The model under review builds one solid part; all positions refer to its coordinate system, in mm. Face numbers are marked on the shaded views. A direction names the side the tool comes from. Round coordinates to 2 decimals unless told otherwise and drop trailing zeros. Loops run counter-clockwise (first coordinate to the right, second up) from the corner with the lowest first, then second, coordinate; pieces in that order, holes last. Notation, with made-up numbers: M 42.25,59 L 51.25,59 A21 ccw 51.25,74 Z; hole C -2,-37 d11. An arc over 180 degrees is marked long. Answer as a JSON object with one key per item and string values. Group by question number.
Item 1: To check wall thickness, follow line 1 (X direction, y = -8, z = 8); line 2 (X direction, y = 37.5, z = 4.25); line 3 (Y direction, x = 5, z = 5.5). State the ranges of each line that lie inside material, in increasing order.
Item 2: Consider section B-B (y = -7). Give the boundary of the cut face in (x, z).
Item 3: Consider section C-C (x = -2). Give the boundary of the cut face in (y, z).
Item 4: Consider section A-A (z = 2.5). Give the boundary of the cut face in (x, y) (1 decimal).
Item 5: Insertion check: P1, Ø1.1, axis at y = -24.75, z = 6.75, coming from the -X side; P2, Ø3, axis at x = 13, z = 4, coming from the +Y side (3 decimals); P3, Ø1.5, axis at x = 2, z = 7.5, coming from the -Y side. Each pin has a flat end and moves straight along its axis. Give the tip position at first contact, or say it passes through.
Item 6: Tool access review of the marked faces 1 and 2: name each direction out of +Z, -Z, +X, -X, +Y, -Y from which nothing blocks a thin tool from reaching the whole face with its end or side.
Item 7: Consider section D-D (x = -38.5). Give the boundary of the cut face in (y, z), and give its area (3 significant figures).
```python
from build123d import *

# Parameters (mm, degrees)
F1_DEPTH      = 12.7
F2_T1_DEPTH   = 19.2753145827
F2_T3_DEPTH   = 26.4979139795
F3_R          = 3.81
F4_R          = 0.5908054237
F5_DEPTH      = 57.15
F5_DEPTH_BACK = 73.914


# Not quite as in the source:
# - a fillet or chamfer that OpenCascade refuses, or shapes differently, is made with other operations: its cross-section is extruded or revolved along the edge and cut away or added


with BuildPart() as f1:
    # F0 (on Top) → F1 (new body)
    with BuildSketch(Plane.XY):
        Polygon((13.5222204362, 66.8438002467), (0, 66.8438002467), (-13.5222204362, 66.8438002467), (-50.4813892832, -30.6380242109), (-47.5520528853, -30.6380242109), (-11.6511627941, 64.052532285), (0, 64.052532285), (11.6511627941, 64.052532285), (47.5520528853, -30.6380242109), (50.4813892832, -30.6380242109), align=None)
    extrude(amount=F1_DEPTH)

    # F2: fillet of radius 1.905 on 4 edges, made by hand

    # F2_s2 → F2_t1 (cut)
    with BuildSketch(Plane.XY.offset(-3.2876572913)):
        with BuildLine():
            ThreePointArc((-47.0858443706, -29.4083738154), (-47.784876456, -30.3007560114), (-48.8671158018, -30.6380242109))
            Line((-48.8671158018, -30.6380242109), (-47.5520528853, -30.6380242109))
            Line((-47.5520528853, -30.6380242109), (-47.0858443706, -29.4083738154))
        make_face()
        with BuildLine():
            ThreePointArc((47.0858443706, -29.4083738154), (47.784876456, -30.3007560114), (48.8671158018, -30.6380242109))
            Line((48.8671158018, -30.6380242109), (47.5520528853, -30.6380242109))
            Line((47.5520528853, -30.6380242109), (47.0858443706, -29.4083738154))
        make_face()
    extrude(amount=F2_T1_DEPTH, mode=Mode.SUBTRACT)

    # F2_s4 → F2_t3 (cut)
    with BuildSketch(Plane.XY.offset(-6.8989569898)):
        with BuildLine():
            ThreePointArc((-47.7218064873, -30.6380242109), (-49.2895382878, -29.8152635568), (-49.5030779186, -28.0576746065))
            Line((-49.5030779186, -28.0576746065), (-50.4813892832, -30.6380242109))
            Line((-50.4813892832, -30.6380242109), (-47.7218064873, -30.6380242109))
        make_face()
        with BuildLine():
            ThreePointArc((49.5030779186, -28.0576746065), (49.2895382878, -29.8152635568), (47.7218064873, -30.6380242109))
            Line((47.7218064873, -30.6380242109), (50.4813892832, -30.6380242109))
            Line((50.4813892832, -30.6380242109), (49.5030779186, -28.0576746065))
        make_face()
    extrude(amount=F2_T3_DEPTH, mode=Mode.SUBTRACT)

    # F3
    f3_edges = [f1.edges().sort_by_distance(p)[0] for p in [
        (13.52222, 66.8438, 6.35),
        (-13.52222, 66.8438, 6.35),
        (-11.651163, 64.052532, 6.35),
        (11.651163, 64.052532, 6.35),
    ]]
    fillet(f3_edges, radius=F3_R)

    # F4 (on Right) → F5 (cut, two sides)
    with BuildSketch(Plane.YZ) as f5_sk:
        with Locations((-24.7479453683, 6.7547173239)):
            Circle(F4_R)
    extrude(amount=-F5_DEPTH, mode=Mode.SUBTRACT)
    extrude(f5_sk.sketch, amount=F5_DEPTH_BACK, mode=Mode.SUBTRACT)


solid = f1.part
```
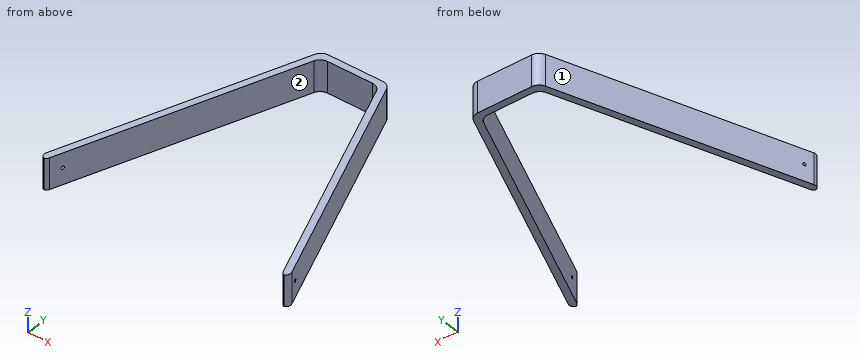
Geometry results:
{
 "1": {"line 1": "x = -41.9 to -38.97, 38.97 to 41.9", "line 2": "x = -24.65 to -21.72, 21.72 to 24.65", "line 3": "y = 64.05 to 66.84"},
 "2": {"outline": "M -41.52,0 L -38.59,0 L -38.59,12.7 L -41.52,12.7 Z; M 38.59,0 L 41.52,0 L 41.52,12.7 L 38.59,12.7 Z"},
 "3": {"outline": "M 64.05,0 L 66.84,0 L 66.84,12.7 L 64.05,12.7 Z"},
 "4": {"outline": "M -49.5,-28.1 A1.9 ccw -48.3,-30.5 A1.9 ccw -47.1,-29.4 L -12.6,61.6 A3.8 cw -9,64.1 L 9,64.1 A3.8 cw 12.6,61.6 L 47.1,-29.4 A1.9 ccw 48.3,-30.5 A1.9 ccw 49.5,-28.1 L 14.5,64.4 A3.8 ccw 10.9,66.8 L -10.9,66.8 A3.8 ccw -14.5,64.4 Z"},
 "5": {"P1": "passes through", "P2": "stops at y = 66.795", "P3": "stops at y = 64.05"},
 "6": {"face 1": "+Z, -Z, -X, +Y", "face 2": "+Z, -Z, -Y"},
 "7": {"outline": "M -6.76,0 L 0.96,0 L 0.96,12.7 L -6.76,12.7 Z", "area": "98.1 mm^2"}
}
